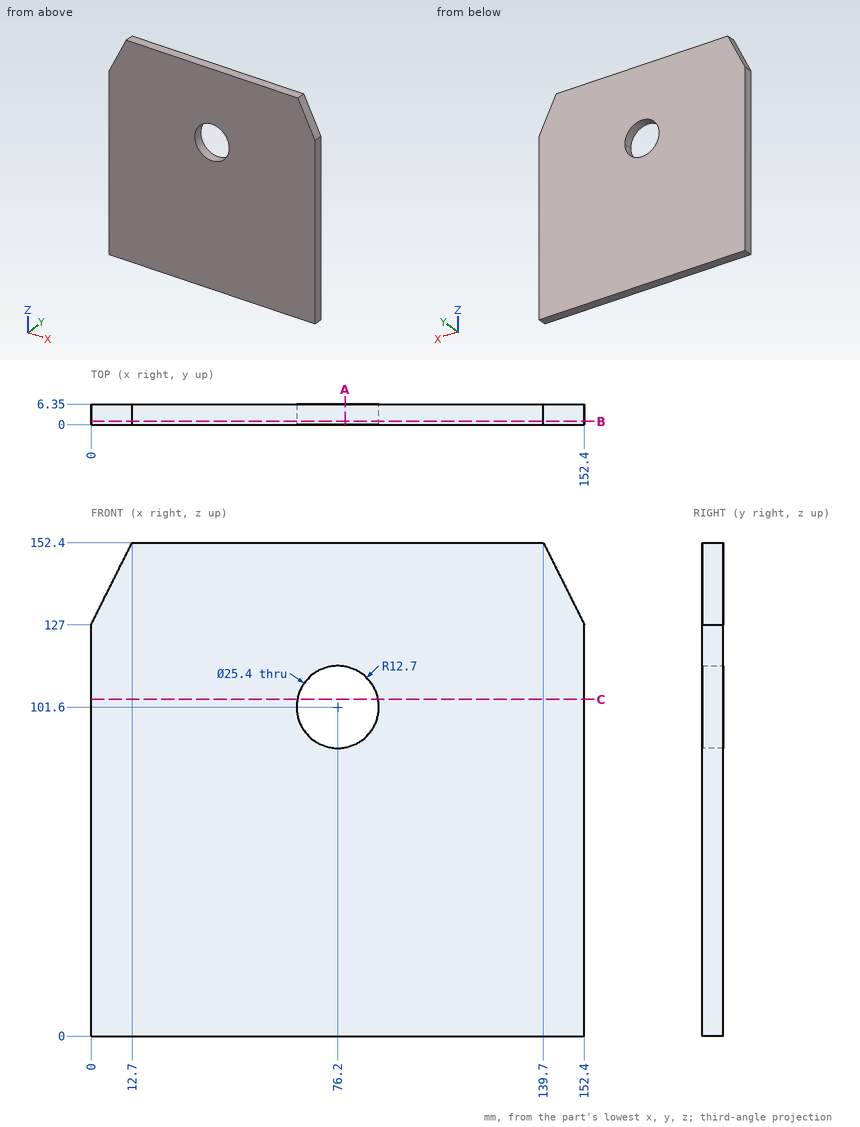
Check sheet for the drawn part. Datum: minimum x, y, z corner. Units: mm. Round coordinates to 2 decimals unless told otherwise and drop trailing zeros. Order: outer loops, then holes, each group sorted by start corner. A loop starts at its lowest first (then second) coordinate and runs counter-clockwise, first axis right, second up. Notation, with made-up numbers: (78, 4) -> (134, 4) arc R8 cw to (134, 12) -> close; hole circle Ø5 at (61, 49.25). An arc over 180 degrees is marked (long way). Put each result on its own line as item: value. Start each with the question number.
(1) Material ranges on line 1 along Z through (x, y) = (76.2, 5.25); line 2 along Z through (x, y) = (66.5, 5.75); line 3 along X through (y, z) = (1, 93), recorded low to high.
(2) Section check B-B (y = 1). Enter the section's corners in (x, z), then the cut area to 3 significant figures.
(3) Section check C-C (z = 104). Enter the section's corners in (x, y).
(4) Section check A-A (x = 78.5). Enter the section's corners in (y, z), then the cut area to 3 significant figures.
Completed:
1. line 1: z = 0 to 88.9, 114.3 to 152.4
1. line 2: z = 0 to 93.4, 109.8 to 152.4
1. line 3: x = 0 to 66.85, 85.55 to 152.4
2. outline: (0, 0) -> (152.4, 0) -> (152.4, 127) -> (139.7, 152.4) -> (12.7, 152.4) -> (0, 127) -> close; hole circle Ø25.4 at (76.2, 101.6)
2. area: 22,400 mm2
3. outline: (0, 0) -> (63.73, 0) -> (63.73, 6.35) -> (0, 6.35) -> close; (88.67, 0) -> (152.4, 0) -> (152.4, 6.35) -> (88.67, 6.35) -> close
4. outline: (0, 0) -> (6.35, 0) -> (6.35, 89.11) -> (0, 89.11) -> close; (0, 114.09) -> (6.35, 114.09) -> (6.35, 152.4) -> (0, 152.4) -> close
4. area: 809 mm2
